from build123d import *

# Parameters (mm, degrees)
F2_W     = 2
F2_H     = 1
F3_DEPTH = 5


with BuildPart() as f1:
    # F0 (on Front) → F1 (revolve)
    with BuildSketch(Plane.XZ):
        Polygon((-3, 1.732051), (0, 0), (0, 20.353371), (-4.5, 20.353371), (-3, 16.732051), align=None)
    revolve(axis=Axis((0, 0, 10.176686), (0, 0, -1)))

    # F2 (on Front) → F3 (cut, symmetric)
    with BuildSketch(Plane.XZ):
        with Locations((0, 19.853371)):
            Rectangle(F2_W, F2_H)
    extrude(amount=F3_DEPTH, both=True, mode=Mode.SUBTRACT)


solid = f1.part
Part model, mm, in its own coordinate system. A direction names the side the tool comes from. Give positions to 0.01 mm unless a question says otherwise; leave off trailing zeros. Order: outer loops, then holes, each group sorted by start corner. A loop starts at its lowest first (then second) coordinate and runs counter-clockwise, first axis right, second up. Notation, with made-up numbers: (-33.5, -6) - (19.5, -6) arc R8 ccw to (19.5, 6) - close; hole circle Ø5 at (19.5, 24). An arc over 180 degrees is marked (long way). Use a Markdown table: item, result.
1) Saw through at A-A on z = 6. List the corners of the cut face in (x, y), plus the area to 3 significant figures.
Checked values:
| item | result |
|---|---|
| outline | circle Ø6 at (0, 0) |
| area | 28.3 mm² |
2) 3-axis set-ups, long thin cutter, end or side, ignore diameter. For faces 1 (the cylindrical face through (3, 0, 9)), 2 (the flat face through (-2, 0, 20.353)), 3 (the flat face through (-1, 0, 20)): which of +Z, -Z, +X, -X, +Y, -Y reach the whole face in a straight line?
Checked values:
| item | result |
|---|---|
| face 1 | -Z |
| face 2 | +Z, +X, -X, +Y, -Y |
| face 3 | +Z, +Y, -Y |
3) Saw through at B-B on z = 18.5. List the corners of the cut face in (x, y), plus the area to 3 significant figures.
Checked values:
| item | result |
|---|---|
| outline | circle Ø7.46 at (0, 0) |
| area | 43.8 mm² |
4) Probe L1, parallel to X at y = 1, z = 9.5; L2, parallel to X at y = -1.5, z = 14. List the from-to ranges inside material, lowest first. Write a range as from..to.
Checked values:
| item | result |
|---|---|
| L1 | -2.83..2.83 |
| L2 | -2.6..2.6 |
5) Two-plate mould, pull along X, no slides. Class faces 4 (the flat face through (0, 0, 19.353)), 5 (the conical face through (0, 0, 0)), 6 (the flat face through (2, 0, 20.353)): +X half, -X half, draft (parallel to the pull), parting line (faces both ways), or undercut.
Checked values:
| item | result |
|---|---|
| face 4 | undercut |
| face 5 | parting line |
| face 6 | draft |
6) Flat gauge pins, fed straight in: P1, Ø0.8, axis at y = 2, z = 19.5, coming from the +X side; P2, Ø5, axis at x = -3, z = 6.5, coming from the +Y side; P3, Ø3, axis at x = -3.5, z = 17, coming from the -Y side. Where does each tip first touch, or does it go through?
Checked values:
| item | result |
|---|---|
| P1 | x = 3.9 |
| P2 | y = 2.96 |
| P3 | y = -2.62 |
